```python
from build123d import *

# Parameters (mm, degrees)
BOSS_EXTRU_1_DEPTH      = 25
ESQUISSE2_R             = 12
ENL_V_MAT_EXTRU_1_DEPTH = 74.654599313
ESQUISSE3_R             = 24
BOSS_EXTRU_2_DEPTH      = 20
ESQUISSE4_R             = 24.5
ESQUISSE4_R_2           = 23
ENL_V_MAT_EXTRU_2_DEPTH = 4
CONG_1_R                = 2


with BuildPart() as part:
    # Esquisse1 → Boss.-Extru.1 (new, symmetric)
    with BuildSketch(Plane.XY):
        with BuildLine():
            Line((0, -30), (45, -30))
            Line((45, -30), (45, 30))
            Line((45, 30), (0, 30))
            ThreePointArc((0, 30), (-30, 0), (0, -30))
        make_face()
    extrude(amount=BOSS_EXTRU_1_DEPTH, both=True)

    # Esquisse2 → Enlèv. mat.-Extru.1 (cut, through all)
    with BuildSketch(Plane.XY.offset(25)):
        Circle(ESQUISSE2_R)
    extrude(amount=-ENL_V_MAT_EXTRU_1_DEPTH, mode=Mode.SUBTRACT)

    # Esquisse3 → Boss.-Extru.2 (add)
    with BuildSketch(Plane(origin=(45, 0, 0), x_dir=(0, 0, -1), z_dir=(1, 0, 0))):
        Circle(ESQUISSE3_R)
    extrude(amount=BOSS_EXTRU_2_DEPTH)

    # Esquisse4 → Enlèv. mat.-Extru.2 (cut)
    with BuildSketch(Plane(origin=(61, 0, 0), x_dir=(0, 0, -1), z_dir=(1, 0, 0))):
        Circle(ESQUISSE4_R)
        Circle(ESQUISSE4_R_2, mode=Mode.SUBTRACT)
    extrude(amount=-ENL_V_MAT_EXTRU_2_DEPTH, mode=Mode.SUBTRACT)

    # Congé1
    cong_1_edges = [part.edges().sort_by_distance(p)[0] for p in [
        (45, 0, 25),
        (45, 0, -25),
        (45, 30, 0),
        (45, -30, 0),
    ]]
    fillet(cong_1_edges, radius=CONG_1_R)


solid = part.part
```
Verification items for the finished model (mm, model axes). A direction names the side the tool comes from. Coordinates: 2 decimals unless noted, no trailing zeros. Loops run counter-clockwise (first coordinate to the right, second up) from the corner with the lowest first, then second, coordinate; pieces in that order, holes last. Notation, with made-up numbers: (61, -15.75) - (90, -15.75) arc R18 cw to (90, -2.75) - close; hole circle Ø4 at (39.25, 82). An arc over 180 degrees is marked (long way). Return JSON: item names as keys, results as strings.
1. Section check A-A, the plane z = 0. Record the boundary of the cut face in (x, y), then the cut area to 3 significant figures.
Established:
{"outline": "(0, -30) - (43, -30) arc R2 ccw to (45, -28) - (45, -24) - (57, -24) - (57, -23) - (61, -23) - (61, -24) - (65, -24) - (65, 24) - (61, 24) - (61, 23) - (57, 23) - (57, 24) - (45, 24) - (45, 28) arc R2 ccw to (43, 30) - (0, 30) arc R30 ccw to start; hole circle Ø24 at (0, 0)", "area": "4,610 mm2"}
2. Tool access check on faces 5 (the cylindrical face through (50.916, 1.055, 23.977)), 6 (the flat face through (45, -25, 0)), 7 (the cylindrical face through (44.43, -18.27, 24.4)), 8 (the cylindrical face through (44.4, -18.27, -24.43)). Record the directions out of +Z, -Z, +X, -X, +Y, -Y that give a thin tool (end or side, any length) a straight path to the whole face; none if there is none.
Established:
{"face 5": "+X", "face 6": "+X, -Y", "face 7": "+Z, +X, -Y", "face 8": "-Z, +X, -Y"}
3. Section check D-D, the plane y = 18.5. Record the boundary of the cut face in (x, z), then the cut area to 3 significant figures.
Established:
{"outline": "(-23.62, -25) - (43, -25) arc R2 ccw to (45, -23) - (45, -15.29) - (57, -15.29) - (57, -13.67) - (61, -13.67) - (61, -15.29) - (65, -15.29) - (65, 15.29) - (61, 15.29) - (61, 13.67) - (57, 13.67) - (57, 15.29) - (45, 15.29) - (45, 23) arc R2 ccw to (43, 25) - (-23.62, 25) - close", "area": "4,030 mm2"}
4. Section check B-B, the plane y = 11. Record the boundary of the cut face in (x, z).
Established:
{"outline": "(-27.91, -25) - (-4.8, -25) - (-4.8, 25) - (-27.91, 25) - close; (4.8, -25) - (43, -25) arc R2 ccw to (45, -23) - (45, -21.33) - (57, -21.33) - (57, -20.2) - (61, -20.2) - (61, -21.33) - (65, -21.33) - (65, 21.33) - (61, 21.33) - (61, 20.2) - (57, 20.2) - (57, 21.33) - (45, 21.33) - (45, 23) arc R2 ccw to (43, 25) - (4.8, 25) - close"}
5. Thickness scan on L1, parallel to Y at x = 0, z = 2; L2, parallel to Z at x = 56, y = -1; L3, parallel to X at y = -6, z = -19. Record the ranges inside material, lowest first.
Established:
{"L1": "y = -30 to -12, 12 to 30", "L2": "z = -23.98 to 23.98", "L3": "x = -29.39 to -10.39, 10.39 to 65"}
6. Mould release check, pull along Y, two halves, no side actions. Record for faces 1 (the cylindrical face through (59.028, 22.804, 2.994)), 2 (the cylindrical face through (44.43, 18.59, 24.4)), 3 (the flat face through (22, 30, 0)), 4 (the cylindrical face through (-11.99, 0.53, 0.35)): +Y half, -Y half, draft (parallel to the pull), parting line (faces both ways), or undercut.
Established:
{"face 1": "parting line", "face 2": "draft", "face 3": "+Y half", "face 4": "undercut"}
7. Go/stop test with flat-tipped pins: pin 1 (6 mm diameter, centred on y = -19, z = -4, fed in from -X); pin 2 (24 mm diameter, centred on y = 10.5, z = 6.5, fed in from -X); pin 3 (2 mm diameter, centred on x = -9, z = 9.5, fed in from +Y); pin 4 (19 mm diameter, centred on x = 0, y = 0, fed in from +Z). Record where each tip stops, or that it passes through.
Established:
{"pin 1": "stops at x = -25.38", "pin 2": "stops at x = -30", "pin 3": "stops at y = 28.91", "pin 4": "passes through"}
8. Section check C-C, the plane x = -6.5. Record the boundary of the cut face in (y, z).
Established:
{"outline": "(-29.29, -25) - (-10.09, -25) - (-10.09, 25) - (-29.29, 25) - close; (10.09, -25) - (29.29, -25) - (29.29, 25) - (10.09, 25) - close"}
